Source: CAD feature listing. Evaluate the final solid. Frame: model axes, mm. Face numbers are marked on the shaded views. A direction names the side the tool comes from. Round coordinates to 2 decimals unless told otherwise and drop trailing zeros. Write each loop counter-clockwise with the first axis right and the second up, starting at its lowest first coordinate (ties: lowest second). Pieces come first, ordered by that corner, then holes. Notation, with made-up numbers: (80.5, 25) -> (113.5, 25) arc R25 cw to (113.5, 47) -> close; hole circle Ø5 at (34.25, 31.25). An arc over 180 degrees is marked (long way). Put each result on its own line as item: value.
```python
from build123d import *

# Parameters (mm, degrees)
F0_R     = 9.5
F0_R_2   = 7.5
F1_DEPTH = 18.5
F2_DEPTH = 16
F3_R     = 3.5
F4_DEPTH = 7.001


with BuildPart() as f1:
    # F0 (on Front) → F1 (new body)
    with BuildSketch(Plane.XZ):
        Circle(F0_R)
        Circle(F0_R_2, mode=Mode.SUBTRACT)
    extrude(amount=F1_DEPTH)

    # F0 (on Front) → F2 (join)
    with BuildSketch(Plane.XZ):
        with BuildLine():
            Line((-40, -22), (0, -22))
            Line((0, -22), (40, -22))
            Line((40, -22), (40, -15))
            Line((40, -15), (21, -15))
            Line((21, -15), (21, 0))
            ThreePointArc((21, 0), (14.849242, 14.849242), (0, 21))
            ThreePointArc((0, 21), (-14.849242, 14.849242), (-21, 0))
            Line((-21, 0), (-21, -15))
            Line((-21, -15), (-40, -15))
            Line((-40, -15), (-40, -22))
        make_face()
        Circle(F0_R, mode=Mode.SUBTRACT)
    extrude(amount=F2_DEPTH)

    # F3 (on face) → F4 (cut, through all)
    with BuildSketch(Plane.XY.offset(-15)):
        with Locations((-31.5, -8)):
            Circle(F3_R)
        with Locations((31.5, -8)):
            Circle(F3_R)
    extrude(amount=-F4_DEPTH, mode=Mode.SUBTRACT)


solid = f1.part
```
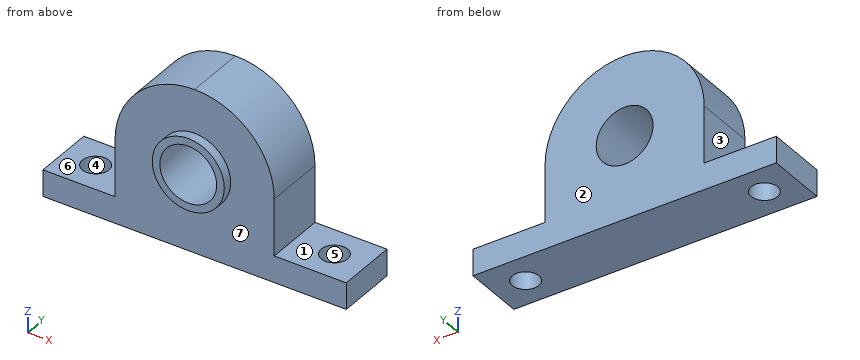
Q1. Draft query along Y for the marked faces 4, 5, 6 and 7. Return one class per face: +Y half, -Y half, draft (parallel to the pull), parting line (faces both ways), or undercut.
Ans:
face 4: undercut
face 5: undercut
face 6: draft
face 7: -Y half
Q2. Reachability of the marked faces 1, 2 and 3 from +Z, -Z, +X, -X, +Y, -Y: full face, straight path, thin tool, end or side. Return the list, or none.
Ans:
face 1: +Z, +X, +Y, -Y
face 2: +Z, -Z, +X, -X, +Y
face 3: +Z, -X, +Y, -Y
Q3. Pin query (flat end, axial travel): pin 1 (5.5 mm diameter, centred on x = 31.5, y = -8, fed in from -Z); pin 2 (5 mm diameter, centred on x = -4, y = -11, fed in from +Z); pin 3 (7.5 mm diameter, centred on y = -12, z = -10, fed in from -X); pin 4 (3 mm diameter, centred on x = 8, z = -8, fed in from -Y). Return the tip coordinate at first contact, or that it passes through.
Ans:
pin 1: passes through
pin 2: stops at z = 20.95
pin 3: stops at x = -21
pin 4: stops at y = -16
Q4. Material intervals for line 1 (Z direction, x = 0, y = -7); line 2 (Y direction, x = 31.5, z = -19); line 3 (X direction, y = -10, z = -16), sorted ascending. Write a range as [from, to].
Ans:
line 1: z = [-22, -7.5], [7.5, 21]
line 2: y = [-16, -11.5], [-4.5, 0]
line 3: x = [-40, -34.37], [-28.63, 28.63], [34.37, 40]
Q5. Cut plane C-C on z = -4. Output: boundary loops of the cut face in (x, y).
Ans:
outline: (-21, -16) -> (-8.62, -16) -> (-8.62, -18.5) -> (-6.34, -18.5) -> (-6.34, 0) -> (-21, 0) -> close; (6.34, -18.5) -> (8.62, -18.5) -> (8.62, -16) -> (21, -16) -> (21, 0) -> (6.34, 0) -> close
Q6. Cut plane A-A on x = -31.5. Output: boundary loops of the cut face in (y, z).
Ans:
outline: (-16, -22) -> (-11.5, -22) -> (-11.5, -15) -> (-16, -15) -> close; (-4.5, -22) -> (0, -22) -> (0, -15) -> (-4.5, -15) -> close
Q7. Cut plane B-B on y = -8. Output: boundary loops of the cut face in (x, z).
Ans:
outline: (-40, -22) -> (-35, -22) -> (-35, -15) -> (-40, -15) -> close; (-28, -22) -> (28, -22) -> (28, -15) -> (21, -15) -> (21, 0) arc R21 ccw to (0, 21) arc R21 ccw to (-21, 0) -> (-21, -15) -> (-28, -15) -> close; (35, -22) -> (40, -22) -> (40, -15) -> (35, -15) -> close; hole circle Ø15 at (0, 0)
Q8. Cut plane D-D on x = 33.5. Output: boundary loops of the cut face in (y, z), and give its area (3 significant figures).
Ans:
outline: (-16, -22) -> (-10.87, -22) -> (-10.87, -15) -> (-16, -15) -> close; (-5.13, -22) -> (0, -22) -> (0, -15) -> (-5.13, -15) -> close
area: 71.8 mm^2
